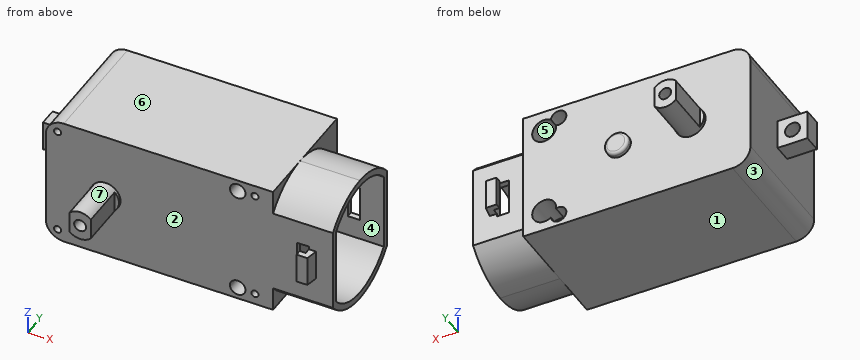
from build123d import *

# Parameters (mm, degrees)
SALIENTE_EXTRUIR1_DEPTH = 10
CROQUIS1_3_W            = 5
CROQUIS1_3_H            = 5
CROQUIS1_3_R            = 1.25
SALIENTE_EXTRUIR2_DEPTH = 1.5
CROQUIS5_R              = 2.5
SALIENTE_EXTRUIR3_DEPTH = 8
CORTAR_EXTRUIR7_START   = -7.5
CORTAR_EXTRUIR7_DEPTH   = 7.5
CROQUIS7_R              = 1
CORTAR_EXTRUIR8_DEPTH   = 36
CORTAR_EXTRUIR18_DEPTH  = 10
CROQUIS9_R              = 1.3
CORTAR_EXTRUIR16_DEPTH  = 36
CROQUIS11_R             = 2
SALIENTE_EXTRUIR4_DEPTH = 1
REDONDEO1_R             = 0.5
CROQUIS12_R             = 0.6
CORTAR_EXTRUIR17_DEPTH  = 9
CROQUIS15_R             = 2
CORTAR_EXTRUIR21_DEPTH  = 5
CROQUIS16_R             = 2.5
CORTAR_EXTRUIR22_DEPTH  = 10
CROQUIS17_W             = 2
CROQUIS17_H             = 6
CORTAR_EXTRUIR23_DEPTH  = 20
SALIENTE_EXTRUIR5_DEPTH = 2.5


with BuildPart() as part:
    # Croquis1 → Saliente-Extruir1 (new, symmetric)
    with BuildSketch(Plane(origin=(0, 0, 0), x_dir=(1, 0, 0), z_dir=(0, 1, 0))):
        with BuildLine():
            ThreePointArc((-24, 8), (-23.121320344, 10.121320344), (-21, 11))
            Line((-21, 11), (24, 11))
            Line((24, 11), (24, -11))
            Line((24, -11), (-21, -11))
            ThreePointArc((-21, -11), (-23.121320344, -10.121320344), (-24, -8))
            Line((-24, -8), (-24, -2.5))
            Line((-24, -2.5), (-24, 2.5))
            Line((-24, 2.5), (-24, 8))
        make_face()
    extrude(amount=SALIENTE_EXTRUIR1_DEPTH, both=True)

    # Croquis1<3> → Saliente-Extruir2 (add, symmetric)
    with BuildSketch(Plane(origin=(0, 0, 0), x_dir=(1, 0, 0), z_dir=(0, 1, 0))):
        with Locations((-26.5, 0)):
            Rectangle(CROQUIS1_3_W, CROQUIS1_3_H)
        with Locations(Location((-26.5, 0, 0), (0, 0, 270))):
            Circle(CROQUIS1_3_R, mode=Mode.SUBTRACT)
    extrude(amount=SALIENTE_EXTRUIR2_DEPTH, both=True)

    # Croquis5 → Saliente-Extruir3 (add)
    with BuildSketch(Plane(origin=(0, 10, 0), x_dir=(1, 0, 0), z_dir=(0, 1, 0))):
        with Locations(Location((-14, 0, 0), (0, 0, 270))):
            Circle(CROQUIS5_R)
    saliente_extruir3 = extrude(amount=SALIENTE_EXTRUIR3_DEPTH)

    # Croquis6 → Cortar-Extruir7 (cut)
    with BuildSketch(Plane(origin=(0, 18, 0), x_dir=(1, 0, 0), z_dir=(0, 1, 0)).offset(CORTAR_EXTRUIR7_START)):
        with BuildLine():
            Line((-15.785357107, 1.75), (-15.785357107, -1.75))
            ThreePointArc((-15.785357107, -1.75), (-16.5, 0), (-15.785357107, 1.75))
        make_face()
        with BuildLine():
            Line((-12.214642893, 1.75), (-12.214642893, -1.75))
            ThreePointArc((-12.214642893, -1.75), (-11.5, 0), (-12.214642893, 1.75))
        make_face()
    cortar_extruir7 = extrude(amount=CORTAR_EXTRUIR7_DEPTH, mode=Mode.SUBTRACT)

    # Simetría2: Saliente-Extruir3, Cortar-Extruir7 across plane
    add(saliente_extruir3.mirror(Plane.ZX))
    add(cortar_extruir7.mirror(Plane.ZX), mode=Mode.SUBTRACT)

    # Croquis7 → Cortar-Extruir8 (cut)
    with BuildSketch(Plane(origin=(0, 18, 0), x_dir=(1, 0, 0), z_dir=(0, 1, 0))):
        with Locations(Location((-14, 0, 0), (0, 0, 270))):
            Circle(CROQUIS7_R)
    extrude(amount=-CORTAR_EXTRUIR8_DEPTH, mode=Mode.SUBTRACT)

    # Croquis13 → Cortar-Extruir18 (cut)
    with BuildSketch(Plane(origin=(24, 0, 0), x_dir=(0, 0, -1), z_dir=(1, 0, 0))):
        with BuildLine():
            Line((-11, 10), (-11, -1.5))
            ThreePointArc((-11, -1.5), (-9.944931378, 3.200887138), (-6.982120022, 7))
            Line((-6.982120022, 7), (6.982120022, 7))
            ThreePointArc((6.982120022, 7), (9.944931392, 3.200887108), (11, -1.500000065))
            Line((11, -1.500000065), (11, 10))
            Line((11, 10), (-11, 10))
        make_face()
        with BuildLine():
            ThreePointArc((11, -1.500000065), (9.944931364, -6.200887167), (6.982120022, -10))
            Line((6.982120022, -10), (11, -10))
            Line((11, -10), (11, -1.500000065))
        make_face()
        with BuildLine():
            Line((0, 6), (-6.5, 6))
            ThreePointArc((-6.5, 6), (-9.924716621, -1.5), (-6.5, -9))
            Line((-6.5, -9), (0, -9))
            Line((0, -9), (0, 6))
        make_face()
        with BuildLine():
            Line((6.5, 6), (0, 6))
            Line((0, 6), (0, -9))
            Line((0, -9), (6.5, -9))
            ThreePointArc((6.5, -9), (9.924716621, -1.5), (6.5, 6))
        make_face()
        with BuildLine():
            Line((-11, -10), (-6.982120022, -10))
            ThreePointArc((-6.982120022, -10), (-9.944931378, -6.200887138), (-11, -1.5))
            Line((-11, -1.5), (-11, -10))
        make_face()
    extrude(amount=-CORTAR_EXTRUIR18_DEPTH, mode=Mode.SUBTRACT)

    # Croquis9 → Cortar-Extruir16 (cut)
    with BuildSketch(Plane(origin=(0, 10, 0), x_dir=(1, 0, 0), z_dir=(0, 1, 0))):
        with Locations(Location((8.091085786, 9, 0), (0, 0, 270))):
            Circle(CROQUIS9_R)
        with Locations(Location((8.091085786, -9, 0), (0, 0, 270))):
            Circle(CROQUIS9_R)
    extrude(amount=-CORTAR_EXTRUIR16_DEPTH, mode=Mode.SUBTRACT)

    # Croquis11 → Saliente-Extruir4 (add)
    with BuildSketch(Plane(origin=(0, 10, 0), x_dir=(1, 0, 0), z_dir=(0, 1, 0))):
        with Locations(Location((-2, 0, 0), (0, 0, 270))):
            Circle(CROQUIS11_R)
    extrude(amount=SALIENTE_EXTRUIR4_DEPTH)

    # Redondeo1
    redondeo1_edges = [part.edges().sort_by_distance(p)[0] for p in [
        (-2, 11, -2),
    ]]
    fillet(redondeo1_edges, radius=REDONDEO1_R)

    # Croquis12 → Cortar-Extruir17 (cut)
    with BuildSketch(Plane.XZ.offset(10)):
        with Locations(Location((-22.030762345, 9.117944486, 0), (0, 0, 270))):
            Circle(CROQUIS12_R)
        with Locations(Location((10.969237655, 9.117944486, 0), (0, 0, 270))):
            Circle(CROQUIS12_R)
        with Locations(Location((10.969237655, -9.117944486, 0), (0, 0, 90))):
            Circle(CROQUIS12_R)
        with Locations(Location((-22.030762345, -9.117944486, 0), (0, 0, 90))):
            Circle(CROQUIS12_R)
    extrude(amount=-CORTAR_EXTRUIR17_DEPTH, mode=Mode.SUBTRACT)

    # Croquis15 → Cortar-Extruir21 (cut)
    with BuildSketch(Plane(origin=(0, 10, 0), x_dir=(1, 0, 0), z_dir=(0, 1, 0))):
        with Locations((10.5, 7.5)):
            Circle(CROQUIS15_R)
        with Locations((10.5, -7.5)):
            Circle(CROQUIS15_R)
    extrude(amount=-CORTAR_EXTRUIR21_DEPTH, mode=Mode.SUBTRACT)

    # Croquis16 → Cortar-Extruir22 (cut)
    with BuildSketch(Plane(origin=(14, 0, 0), x_dir=(0, 0, -1), z_dir=(1, 0, 0))):
        with Locations((0, -1.5)):
            Circle(CROQUIS16_R)
    extrude(amount=-CORTAR_EXTRUIR22_DEPTH, mode=Mode.SUBTRACT)

    # Croquis17 → Cortar-Extruir23 (cut)
    with BuildSketch(Plane(origin=(0, 7, 0), x_dir=(1, 0, 0), z_dir=(0, 1, 0))):
        with Locations((19, 0.002120022)):
            Rectangle(CROQUIS17_W, CROQUIS17_H)
    extrude(amount=-CORTAR_EXTRUIR23_DEPTH, mode=Mode.SUBTRACT)

    # Croquis18 → Saliente-Extruir5 (add, symmetric)
    with BuildSketch(Plane.XY):
        Polygon((21.2, 7), (20.8, 9), (19, 9), (19, 8), (20, 8), (20, 7), align=None)
    saliente_extruir5 = extrude(amount=SALIENTE_EXTRUIR5_DEPTH, both=True)

    # Simetría3: Saliente-Extruir5 across plane
    add(saliente_extruir5.mirror(Plane.ZX.offset(-1.5)))


solid = part.part
Input: part model. Units: mm. Frame: model coordinates. Face numbers are marked on the shaded views. A direction names the side the tool comes from. Round coordinates to 2 decimals unless told otherwise and drop trailing zeros. Order: outer loops, then holes, each group sorted by start corner. A loop starts at its lowest first (then second) coordinate and runs counter-clockwise, first axis right, second up. Notation, with made-up numbers: (-35, 12.5) - (22, 12.5) arc R9 cw to (22, 24.5) - close; hole circle Ø10 at (8, 88.25). An arc over 180 degrees is marked (long way). Answer as a JSON object with one key per item and string values. Group by question number.
(1) Material intervals for probe 1 along Y at (x, z) = (15, -2); probe 2 along Y at (x, z) = (9.75, 0); probe 3 along Z at (x, y) = (9, -1), sorted ascending. Write a range as from..to.
(2) Reachability of the marked faces 4, 5, 6 and 7 from +Z, -Z, +X, -X, +Y, -Y: full face, straight path, thin tool, end or side. Return the list, or none.
(3) Cut plane C-C (x = -14). Return loops of the section in (y, z), then the cut area to 3 significant figures.
(4) Draft query along X for the marked faces 1, 2 and 3. Return one class per face: released by +X, released by -X, zero draft, split by the parting line, or undercut.
(5) Cut plane B-B (y = -14). Return loops of the section in (x, z).
(6) Cut plane A-A (x = -26.5). Return loops of the section in (y, z), then the cut area to 3 significant figures.
(7) Pin query (flat end, axial travel): P1, Ø3, axis at y = -6.5, z = 3, coming from the +X side; P2, Ø0.6, axis at x = 11, z = -9.5, coming from the -Y side; P3, Ø3.5, axis at x = -2, z = 0, coming from the +Y side. Return the tip coordinate at first contact, or that it passes through.
Here are the results:
{
 "1": {"probe 1": "y = -10..-9, 6..7", "probe 2": "y = -10..-4, 1..10", "probe 3": "z = -11..-9.93, -8.07..-2.45, 2.45..8.07, 9.93..11"},
 "2": {"face 4": "+X", "face 5": "+Y", "face 6": "+Z, +X, -X, +Y, -Y", "face 7": "-Y"},
 "3": {"outline": "(-18, -2.5) - (-10, -2.5) - (-10, -11) - (10, -11) - (10, -2.5) - (18, -2.5) - (18, -1) - (-18, -1) - close; (-18, 1) - (18, 1) - (18, 2.5) - (10, 2.5) - (10, 11) - (-10, 11) - (-10, 2.5) - (-18, 2.5) - close", "area": "448 mm^2"},
 "4": {"face 1": "zero draft", "face 2": "undercut", "face 3": "released by -X"},
 "5": {"outline": "(-15.79, -1.75) arc R2.5 ccw to (-12.21, -1.75) - (-12.21, 1.75) arc R2.5 ccw to (-15.79, 1.75) - close; hole circle Ø2 at (-14, 0)"},
 "6": {"outline": "(-1.5, -2.5) - (1.5, -2.5) - (1.5, -1.25) - (-1.5, -1.25) - close; (-1.5, 1.25) - (1.5, 1.25) - (1.5, 2.5) - (-1.5, 2.5) - close", "area": "7.50 mm^2"},
 "7": {"P1": "stops at x = 14", "P2": "stops at y = -10", "P3": "stops at y = 11"}
}
